from build123d import *

# Parameters (mm, degrees)
F0_W     = 52.07
F0_H     = 52.07
F1_DEPTH = 12.7
F2_W     = 52.07
F2_H     = 6.35
F3_DEPTH = 6.35
F4_W     = 12.7
F4_H     = 6.35
F5_DEPTH = 3.302


with BuildPart() as f1:
    # F0 (on Top) → F1 (new body)
    with BuildSketch(Plane.XY):
        Polygon((41.3333964217, 37.3389664483), (-17.0866035783, 37.3389664483), (-23.4366035783, 37.3389664483), (-23.4366035783, -27.4310335517), (41.3333964217, -27.4310335517), align=None)
        with Locations((8.9483964217, 4.9539664483)):
            Rectangle(F0_W, F0_H, mode=Mode.SUBTRACT)
    extrude(amount=F1_DEPTH)

    # F2 (on face) → F3 (cut)
    with BuildSketch(Plane.XY.offset(12.7)):
        with Locations((8.9483964217, 34.1639664483)):
            Rectangle(F2_W, F2_H)
        with Locations((8.9483964217, -24.2560335517)):
            Rectangle(F2_W, F2_H)
    extrude(amount=-F3_DEPTH, mode=Mode.SUBTRACT)

    # F4 (on face) → F5 (cut)
    with BuildSketch(Plane.XY.offset(6.35)):
        with Locations((28.6333964217, -24.2560335517)):
            Rectangle(F4_W, F4_H)
    extrude(amount=-F5_DEPTH, mode=Mode.SUBTRACT)


solid = f1.part
Geometry check sheet. Reference: the model listing, model coordinates, mm. A direction names the side the tool comes from. Round coordinates to 2 decimals unless told otherwise and drop trailing zeros. Loops run counter-clockwise (first coordinate to the right, second up) from the corner with the lowest first, then second, coordinate; pieces in that order, holes last. Notation, with made-up numbers: (-24, 52.5) - (-19, 52.5) arc R21 ccw to (-19, 60.5) - close; hole circle Ø3 at (58.5, -0.5). An arc over 180 degrees is marked (long way). One line per question, with ' | ' between items. Start each with the question number.
1. Scan lines: line 1 (X direction, y = 1, z = 12); line 2 (Y direction, x = -3, z = 5.25); line 3 (Z direction, x = 34, y = -22). Record each from-to range of solid material in increasing order. Write a range as [from, to].
2. Cross-section at A-A on x = -5. Record the cut outline in (y, z), then the cut area to 3 significant figures.
3. Tool access check on faces 4 (the face through (-17.087, 5, 6)), 5 (the face through (38, 5, 12.7)), 6 (the face through (2, -24, 6.35)), 7 (the face through (22.283, -24, 5)), 8 (the face through (9, -21.081, 3)). Record the directions out of +Z, -Z, +X, -X, +Y, -Y that give a thin tool (end or side, any length) a straight path to the whole face; none if there is none.
4. Draft check along X on faces 1 (the face through (41.333, 5, 6)), 2 (the face through (9, 34, 6.35)), 3 (the face through (8, -23, 0)). Enter one of: released by +X, released by -X, zero draft, split by the parting line, or undercut.
5. Cross-section at C-C on y = 32. Record the cut outline in (x, z), then the cut area to 3 significant figures.
6. Cross-section at B-B on z = 11. Record the cut outline in (x, y), then the cut area to 3 significant figures.
7. Cross-section at D-D on z = 5.25. Record the cut outline in (x, y), then the cut area to 3 significant figures.
8. Depth check by flat-ended pin: pin 1 (1.9 mm diameter, centred on x = -1.5, y = 33.5, fed in from +Z). Enter the tip coordinate at first touch or a pass-through.
Taken from the geometry:
1) line 1: [-23.44, -17.09], [34.98, 41.33] | line 2: [-27.43, -21.08], [30.99, 37.34] | line 3: [0, 3.05]
2) outline: (-27.43, 0) - (-21.08, 0) - (-21.08, 6.35) - (-27.43, 6.35) - close; (30.99, 0) - (37.34, 0) - (37.34, 6.35) - (30.99, 6.35) - close | area: 80.6 mm²
3) face 4: +Z | face 5: +Z, +X, -X, +Y, -Y | face 6: +Z, +Y, -Y | face 7: +Z, -Y | face 8: +Z, -Z
4) face 1: released by +X | face 2: undercut | face 3: zero draft
5) outline: (-23.44, 0) - (41.33, 0) - (41.33, 12.7) - (34.98, 12.7) - (34.98, 6.35) - (-17.09, 6.35) - (-17.09, 12.7) - (-23.44, 12.7) - close | area: 492 mm²
6) outline: (-23.44, -27.43) - (-17.09, -27.43) - (-17.09, 37.34) - (-23.44, 37.34) - close; (34.98, -27.43) - (41.33, -27.43) - (41.33, 37.34) - (34.98, 37.34) - close | area: 823 mm²
7) outline: (-23.44, -27.43) - (22.28, -27.43) - (22.28, -21.08) - (-17.09, -21.08) - (-17.09, 30.99) - (34.98, 30.99) - (34.98, -27.43) - (41.33, -27.43) - (41.33, 37.34) - (-23.44, 37.34) - close | area: 1,400 mm²
8) pin 1: z = 6.35
